Geometry: final body of the model. Coordinates: model frame, mm. Face numbers are marked on the shaded views. Coordinates: 2 decimals unless noted, no trailing zeros. Loops run counter-clockwise (first coordinate to the right, second up) from the corner with the lowest first, then second, coordinate; pieces in that order, holes last. Notation, with made-up numbers: (84, 61) - (126, 61) arc R25 ccw to (126, 79) - close; hole circle Ø3 at (-21.5, 39). An arc over 180 degrees is marked (long way). Answer in a Markdown table with one row per item.
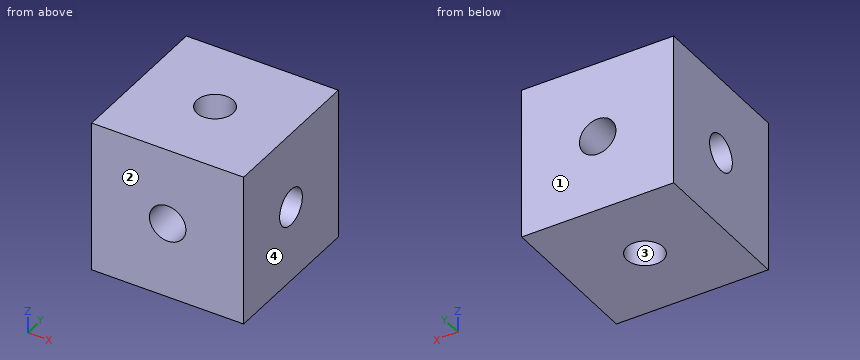
from build123d import *

# Parameters (mm, degrees)
SKETCH_1_W          = 10
SKETCH_1_H          = 10
SKETCH_1_R          = 1.2
EXTRUDE_1_DEPTH     = 10
SKETCH_2_R          = 1.2
CUT_EXTRUDE_1_DEPTH = 18.320508076
SKETCH_3_R          = 1.2
CUT_EXTRUDE_2_DEPTH = 10


with BuildPart() as part:
    # 草图1 → 凸台-拉伸1 (new body)
    with BuildSketch(Plane.XY):
        with Locations((5, 5)):
            Rectangle(SKETCH_1_W, SKETCH_1_H)
        with Locations((5, 5)):
            Circle(SKETCH_1_R, mode=Mode.SUBTRACT)
    extrude(amount=EXTRUDE_1_DEPTH)

    # 草图2 → 切除-拉伸1 (cut, through all)
    with BuildSketch(Plane(origin=(0, 10, 0), x_dir=(1, 0, 0), z_dir=(0, 1, 0))):
        with Locations(Location((5, -5, 0), (0, 0, 180))):
            Circle(SKETCH_2_R)
    extrude(amount=-CUT_EXTRUDE_1_DEPTH, mode=Mode.SUBTRACT)

    # 草图3 → 切除-拉伸2 (cut)
    with BuildSketch(Plane(origin=(10, 0, 0), x_dir=(0, 0, -1), z_dir=(1, 0, 0))):
        with Locations((-5, 5)):
            Circle(SKETCH_3_R)
    extrude(amount=-CUT_EXTRUDE_2_DEPTH, mode=Mode.SUBTRACT)


solid = part.part
(1) Cut plane C-C on x = 2.5. Output: boundary loops of the cut face in (y, z).
Verdict:
| item | result |
|---|---|
| outline | (0, 0) - (10, 0) - (10, 10) - (0, 10) - close; hole circle Ø2.4 at (5, 5) |
(2) Cut plane A-A on y = 5. Output: boundary loops of the cut face in (x, z), then the cut area to 3 significant figures.
Verdict:
| item | result |
|---|---|
| outline | (0, 0) - (3.8, 0) - (3.8, 3.8) - (0, 3.8) - close; (0, 6.2) - (3.8, 6.2) - (3.8, 10) - (0, 10) - close; (6.2, 0) - (10, 0) - (10, 3.8) - (6.2, 3.8) - close; (6.2, 6.2) - (10, 6.2) - (10, 10) - (6.2, 10) - close |
| area | 57.8 mm² |
(3) Pull-direction query (Y, two-part tool) for the marked faces 1, 2, 3 and 4; classes: pulls with the +Y half, pulls with the -Y half, needs draft (parallel to the pull), parting line crosses it, or undercut.
Verdict:
| item | result |
|---|---|
| face 1 | pulls with the +Y half |
| face 2 | pulls with the -Y half |
| face 3 | undercut |
| face 4 | needs draft |
(4) Ray query, probe 1 along Y at (x, z) = (8.3, 5). Return the intervals inside material, ascending.
Verdict:
| item | result |
|---|---|
| probe 1 | y = 0 to 3.8, 6.2 to 10 |
(5) First-contact query: pin 1 Ø3 at (y, z) = (5, 5) entering from -X. Flat tip, straight axial feed; report the tip coordinate or a pass-through.
Verdict:
| item | result |
|---|---|
| pin 1 | stops at x = 0 |
